Verification items for the finished model (mm, model axes). A direction names the side the tool comes from. Round coordinates to 2 decimals unless told otherwise and drop trailing zeros. Write each loop counter-clockwise with the first axis right and the second up, starting at its lowest first coordinate (ties: lowest second). Pieces come first, ordered by that corner, then holes. Notation, with made-up numbers: (13.25, 74.25) - (71.25, 74.25) arc R20 ccw to (71.25, 97.25) - close; hole circle Ø7 at (43.5, 45). An arc over 180 degrees is marked (long way). Answer as a JSON object with one key per item and string values. Group by question number.
1) Section check B-B (z = 14). Enter the section's corners in (x, y).
2) Section check A-A (x = 5.5). Enter the section's corners in (y, z), then the cut area to 4 significant figures.
3) Section check C-C (y = -13). Enter the section's corners in (x, z).
4) Mould release check, pull along Z, two halves, no side actions. Record for faces 1 (the flat face through (10, -15.226, -16)), 2 (the flat face through (13, -16.022, -42)), 3 (the flat face through (46, -13, -60.1)): +Z half, -Z half, draft (parallel to the pull), parting line (faces both ways), or undercut.
5) Go/stop test with flat-tipped pins: pin 1 Ø2.5 at (x, y) = (16.5, -70) entering from +Z; pin 2 Ø3 at (x, z) = (21, -1.5) entering from -Y; pin 3 Ø8 at (y, z) = (-38.5, -27.5) entering from -X; pin 4 Ø12 at (y, z) = (-62, -5) entering from -X. Record where each tip stops, or that it passes through.
6) Thickness scan on line 1 (X direction, y = 20.5, z = -50); line 2 (Y direction, x = 6, z = -16); line 3 (Y direction, x = 50.5, z = 29.5). Record the ranges inside material, lowest first.
7) Set-up check for faces 4 (the flat face through (38, 54.016, -12)), 5 (the flat face through (13, -28, -25.839)), 6 (the flat face through (10, 18, 28.8)), 7 (the flat face through (35.859, -68, -12)): record each of +Z, -Z, +X, -X, +Y, -Y from which the full face is reachable in a straight line by a thin tool's end or side.
8) Section check D-D (z = 25.5). Enter the section's corners in (x, y), then the cut area to 3 significant figures.
```python
from build123d import *

# Parameters (mm, degrees)
F0_W      = 109.69113186
F0_H      = 96.6019369662
F1_DEPTH  = 76.2
F3_DEPTH  = 25.4
F4_W      = 12.1712684631
F4_H      = 10.9790135175
F4_W_2    = 8.8049545884
F4_H_2    = 8.5344947875
F4_W_3    = 9.7688166425
F4_H_3    = 7.8319623135
F4_W_4    = 10.1457694545
F4_H_4    = 9.9510354921
F5_DEPTH  = 12.7
F7_W      = 24.5119724423
F7_H      = 31.4762387425
F8_DEPTH  = 25.4
F9_W      = 15.9004002785
F9_H      = 66.7022062786
F10_DEPTH = 88.9


with BuildPart() as f1:
    # F0 (on Right) → F1 (new body)
    with BuildSketch(Plane.YZ):
        with Locations((-0.8295942098, -11.7987114936)):
            Rectangle(F0_W, F0_H)
    extrude(amount=F1_DEPTH)

    # F2 (on face) → F3 (join)
    with BuildSketch(Plane.XZ.offset(55.6751601398)):
        Polygon((76.2, -60.0996799767), (76.2, 18.9372822642), (57.0150315762, 18.9372822642), (57.0150315762, 0), (35.8594097197, 0), (35.8594097197, -24.5528668165), (18.9174246043, -24.5528668165), (18.9174246043, -46.6084964573), (9.9709145725, -46.6084964573), (9.9709145725, -60.0996799767), align=None)
    extrude(amount=F3_DEPTH)

    # F4 (on face) → F5 (cut)
    with BuildSketch(Plane(origin=(0, 0, 0), x_dir=(0, -1, 0), z_dir=(-1, 0, 0))):
        with Locations((-33.0719724298, 15.969437547)):
            Rectangle(F4_W, F4_H)
        with Locations((-33.8424704969, 0.289965421)):
            Rectangle(F4_W_2, F4_H_2)
        with Locations((-18.260889221, -0.4326736089)):
            Rectangle(F4_W_3, F4_H_3)
        with Locations((-18.0477141403, 15.3193497099)):
            Rectangle(F4_W_4, F4_H_4)
    extrude(amount=-F5_DEPTH, mode=Mode.SUBTRACT)

    # F7 (on face) → F8 (cut)
    with BuildSketch(Plane(origin=(0, 0, 0), x_dir=(0, -1, 0), z_dir=(-1, 0, 0))):
        with Locations((28.2782753929, -41.5770960972)):
            Rectangle(F7_W, F7_H)
    extrude(amount=-F8_DEPTH, mode=Mode.SUBTRACT)

    # F9 (on face) → F10 (cut)
    with BuildSketch(Plane(origin=(0, 0, -60.0996799767), x_dir=(1, 0, 0), z_dir=(0, 0, -1))):
        with Locations((10.4902001393, -18.1248685809)):
            Rectangle(F9_W, F9_H)
    extrude(amount=-F10_DEPTH, mode=Mode.SUBTRACT)


solid = f1.part
```
Returned:
{
 "1": {"outline": "(0, -55.68) - (57.02, -55.68) - (57.02, -81.08) - (76.2, -81.08) - (76.2, 54.02) - (0, 54.02) - (0, 39.16) - (2.54, 39.16) - (2.54, 51.48) - (18.44, 51.48) - (18.44, -15.23) - (2.54, -15.23) - (2.54, 12.97) - (0, 12.97) - close; (0, 23.12) - (2.54, 23.12) - (2.54, 26.99) - (0, 26.99) - close"},
 "2": {"outline": "(-55.68, -60.1) - (-15.23, -60.1) - (-15.23, 28.8) - (51.48, 28.8) - (51.48, -60.1) - (54.02, -60.1) - (54.02, 36.5) - (-55.68, 36.5) - close; hole (-40.53, -57.32) - (-16.02, -57.32) - (-16.02, -25.84) - (-40.53, -25.84) - close", "area": "3,895 mm2"},
 "3": {"outline": "(0, -60.1) - (2.54, -60.1) - (2.54, 28.8) - (18.44, 28.8) - (18.44, -60.1) - (76.2, -60.1) - (76.2, 36.5) - (0, 36.5) - close"},
 "4": {"face 1": "draft", "face 2": "undercut", "face 3": "-Z half"},
 "5": {"pin 1": "z = -46.61", "pin 2": "y = -55.68", "pin 3": "x = 0", "pin 4": "x = 35.86"},
 "6": {"line 1": "0 to 2.54, 18.44 to 76.2", "line 2": "-55.68 to -15.23, 51.48 to 54.02", "line 3": "-55.68 to 54.02"},
 "7": {"face 4": "+Z, -Z, +X, -X, +Y", "face 5": "-X", "face 6": "-Z", "face 7": "+Z, -X, -Y"},
 "8": {"outline": "(0, -55.68) - (76.2, -55.68) - (76.2, 54.02) - (0, 54.02) - close; hole (2.54, -15.23) - (18.44, -15.23) - (18.44, 51.48) - (2.54, 51.48) - close", "area": "7,300 mm2"}
}
